Read the model definition and answer for the solid it produces. Units are mm, in the model's axes. A direction names the side the tool comes from. Coordinates: 2 decimals unless noted, no trailing zeros. Write each loop counter-clockwise with the first axis right and the second up, starting at its lowest first coordinate (ties: lowest second). Pieces come first, ordered by that corner, then holes. Notation, with made-up numbers: (27.25, 14) -> (47.25, 14) arc R13 ccw to (47.25, 34) -> close; hole circle Ø11 at (11.25, -30.5). An arc over 180 degrees is marked (long way). Use CSV: the item, a comma, the result in double quotes.
from build123d import *

# Parameters (mm, degrees)
SKETCH1_R      = 1.5875
EXTRUDE1_DEPTH = 7.4295
SKETCH2_W      = 0.508
SKETCH2_H      = 0.381


with BuildPart() as part:
    # Sketch1 → Extrude1 (new, symmetric)
    with BuildSketch(Plane(origin=(0, 0, 0), x_dir=(0, 0, -1), z_dir=(1, 0, 0))):
        Circle(SKETCH1_R)
    extrude(amount=EXTRUDE1_DEPTH, both=True)

    # Sketch2 → Cut-Revolve1 (revolve, cut)
    with BuildSketch(Plane.XY, mode=Mode.PRIVATE) as cut_revolve1_sk:
        with Locations((-6.4135, 1.397)):
            Rectangle(SKETCH2_W, SKETCH2_H)
        with Locations((6.4135, 1.397)):
            Rectangle(SKETCH2_W, SKETCH2_H)
    revolve(cut_revolve1_sk.sketch.rotate(Axis((-7.4295, 0, 0), (1, 0, 0)), 90), axis=Axis((-7.4295, 0, 0), (1, 0, 0)), mode=Mode.SUBTRACT)


solid = part.part
1. Find the intervals of material crossed by line 1 along X through (y, z) = (1.25, -0.5); line 2 along Y through (x, z) = (0.25, -0.1); line 3 along Y through (x, z) = (0, 0.45), in increasing order.
Solutions:
line 1,"x = -7.43 to -6.67, -6.16 to 6.16, 6.67 to 7.43"
line 2,"y = -1.58 to 1.58"
line 3,"y = -1.52 to 1.52"
2. A tool of negligible diameter and unlimited length cuts with its end or side. For faces 1 (the cylindrical face through (7.05, -1.55, 0.34)), 2 (the flat face through (6.159, -1, -1)), from which of +Z, -Z, +X, -X, +Y, -Y can it reach the whole face along a straight path? Write none if from no direction.
Solutions:
face 1,"+X, -X"
face 2,"none"
3. A cutting plane is placed at C-C (x = -2.25). Give the vertices of the cut face in (y, z) (1 decimal), and give its area (3 significant figures).
Solutions:
outline,"circle Ø3.2 at (0, 0)"
area,"7.92 mm^2"
4. A cutting plane is placed at A-A (y = 0). Give the vertices of the cut face in (x, z), and give its area (3 significant figures).
Solutions:
outline,"(-7.43, -1.59) -> (-6.67, -1.59) -> (-6.67, -1.21) -> (-6.16, -1.21) -> (-6.16, -1.59) -> (6.16, -1.59) -> (6.16, -1.21) -> (6.67, -1.21) -> (6.67, -1.59) -> (7.43, -1.59) -> (7.43, 1.59) -> (6.67, 1.59) -> (6.67, 1.21) -> (6.16, 1.21) -> (6.16, 1.59) -> (-6.16, 1.59) -> (-6.16, 1.21) -> (-6.67, 1.21) -> (-6.67, 1.59) -> (-7.43, 1.59) -> close"
area,"46.4 mm^2"
5. This flat-tipped pin is pushed along its axis until it touches: pin 1 Ø1 at (x, z) = (5.5, -1) entering from +Y. Where does it stop, or does it pass through?
Solutions:
pin 1,"stops at y = 1.51"
